Geometry check sheet. Reference: drawing and pictorial views, mm from the part's lowest x, y, z. Coordinates: 2 decimals unless noted, no trailing zeros. Write each loop counter-clockwise with the first axis right and the second up, starting at its lowest first coordinate (ties: lowest second). Pieces come first, ordered by that corner, then holes. Notation, with made-up numbers: (4.5, 13.25) -> (53.5, 13.25) arc R20 ccw to (53.5, 33.25) -> close; hole circle Ø6 at (28.25, 62). An arc over 180 degrees is marked (long way). Answer in a Markdown table with one row per item.
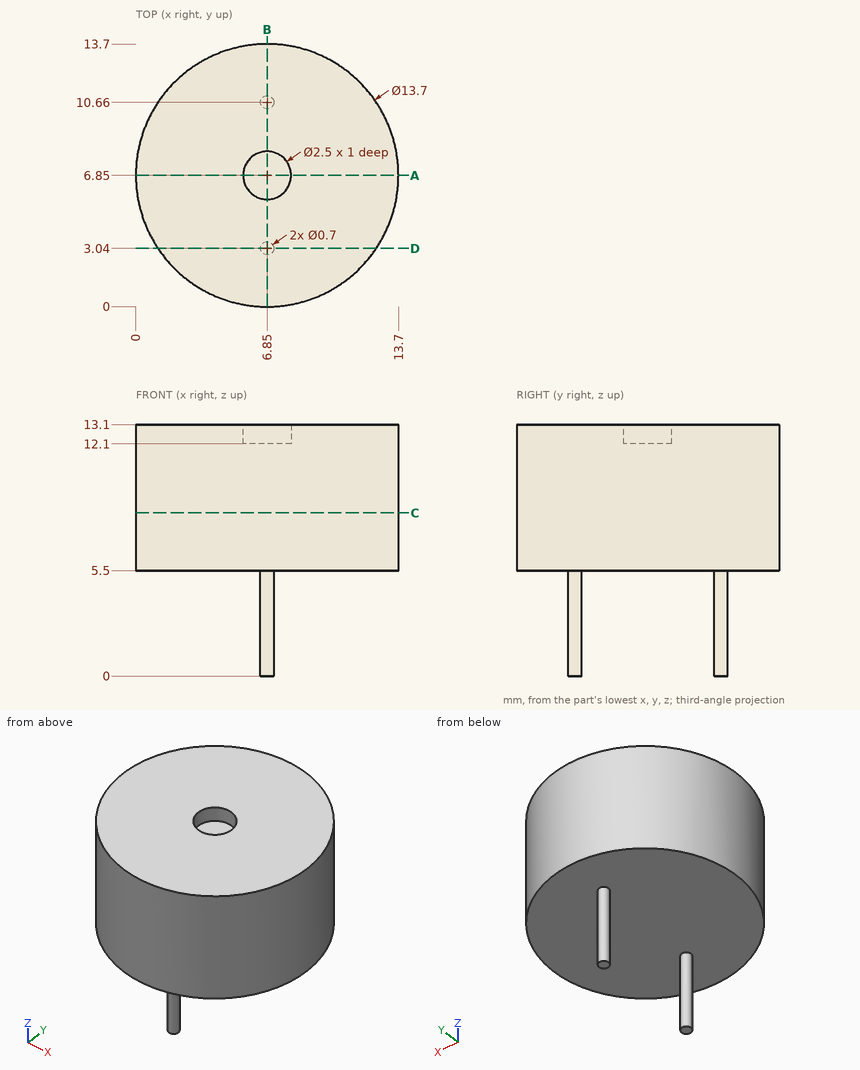
1. Section check B-B, the plane x = 6.85. Record the boundary of the cut face in (y, z), plus the area to 3 significant figures.
Geometry says:
| item | result |
|---|---|
| outline | (0, 5.5) -> (2.69, 5.5) -> (2.69, 0) -> (3.39, 0) -> (3.39, 5.5) -> (10.31, 5.5) -> (10.31, 0) -> (11.01, 0) -> (11.01, 5.5) -> (13.7, 5.5) -> (13.7, 13.1) -> (8.1, 13.1) -> (8.1, 12.1) -> (5.6, 12.1) -> (5.6, 13.1) -> (0, 13.1) -> close |
| area | 109 mm^2 |
2. Section check C-C, the plane z = 8.5. Record the boundary of the cut face in (x, y), plus the area to 3 significant figures.
Geometry says:
| item | result |
|---|---|
| outline | circle Ø13.7 at (6.85, 6.85) |
| area | 147 mm^2 |
3. Thickness scan on line 1 (Y direction, x = 6.85, z = 12.5); line 2 (Z direction, x = 7.75, y = 8.5); line 3 (Y direction, x = 1, z = 9.75). Record the ranges inside material, lowest first. Write a range as from..to.
Geometry says:
| item | result |
|---|---|
| line 1 | 0..5.6, 8.1..13.7 |
| line 2 | 5.5..13.1 |
| line 3 | 3.29..10.41 |
4. Depth check by flat-ended pin: P1, Ø4, axis at x = 5.5, z = 5, coming from the -Y side; P2, Ø4, axis at x = 9, y = 5, coming from the -Z side; P3, Ø2, axis at x = 6.85, y = 6.85, coming from the +Z side. Enter the tip coordinate at first touch or a pass-through.
Geometry says:
| item | result |
|---|---|
| P1 | y = 0 |
| P2 | z = 5.5 |
| P3 | z = 12.1 |
5. Section check A-A, the plane y = 6.85. Record the boundary of the cut face in (x, z), plus the area to 3 significant figures.
Geometry says:
| item | result |
|---|---|
| outline | (0, 5.5) -> (13.7, 5.5) -> (13.7, 13.1) -> (8.1, 13.1) -> (8.1, 12.1) -> (5.6, 12.1) -> (5.6, 13.1) -> (0, 13.1) -> close |
| area | 102 mm^2 |
6. Section check D-D, the plane y = 3.04. Record the boundary of the cut face in (x, z).
Geometry says:
| item | result |
|---|---|
| outline | (1.16, 5.5) -> (6.5, 5.5) -> (6.5, 0) -> (7.2, 0) -> (7.2, 5.5) -> (12.54, 5.5) -> (12.54, 13.1) -> (1.16, 13.1) -> close |
